Input: part model. Units: mm. Frame: model coordinates. Coordinates: 2 decimals unless noted, no trailing zeros. Loops run counter-clockwise (first coordinate to the right, second up) from the corner with the lowest first, then second, coordinate; pieces in that order, holes last. Notation, with made-up numbers: M 13,86.25 L 18,86.25 A28 cw 18,118.25 Z; hole C 61,38.5 d4. An arc over 180 degrees is marked long. Use a Markdown table: item, result. Add a question column.
1. Section A-A on y = 6.5. Output: boundary loops of the cut face in (x, z).
2. Section C-C on y = -4. Output: boundary loops of the cut face in (x, z).
3. Section B-B on x = -10.5. Output: boundary loops of the cut face in (y, z), then the cut area to 3 significant figures.
4. Pin query (flat end, axial travel): pin 1 (1.5 mm diameter, centred on x = 27, z = 0.5, fed in from +Y); pin 2 (1.5 mm diameter, centred on x = 27.5, z = 1, fed in from -Y); pin 3 (1.5 mm diameter, centred on y = -31, z = 2.5, fed in from -X); pin 4 (1.3 mm diameter, centred on x = 10.5, y = 0, fed in from -Z). Return the tip coordinate at first contact, or that it passes through.
5. Line query: L1, parallel to Y at x = -22.6, z = 1.95; L2, parallel to Y at x = 10.5, z = 0.95; L3, parallel to Y at x = -4, z = 2.9. Output: solid intervals per line, ascending. Write a range as [from, to].
6. Section D-D on y = -38.5. Output: boundary loops of the cut face in (x, z).
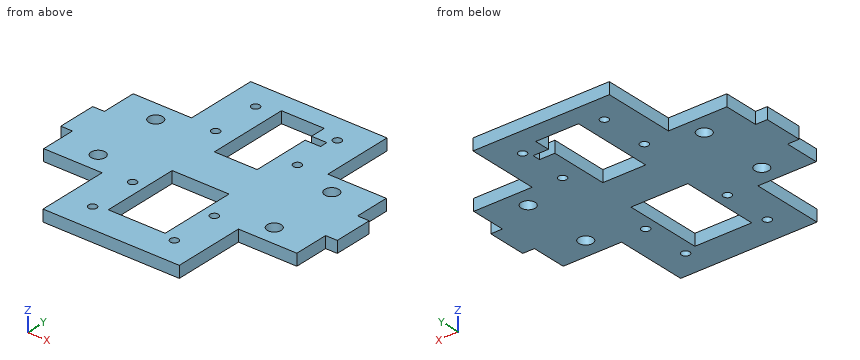
Autodesk Inventor part; units mm, degrees
ref_plane "YZ Plane" through (0, 0, 0) normal (1, 0, 0) x (0, 1, 0)
ref_plane "XZ Plane" through (0, 0, 0) normal (0, 1, 0) x (-1, 0, 0)
ref_plane "XY Plane" through (0, 0, 0) normal (0, 0, 1) x (1, 0, 0)
sketch "Sketch1" plane through (0, 0, 0) normal (0, 0, 1) x (1, 0, 0)
  line L0 (-17.5, 19.5) -> (17.5, 19.5)
  line L1 (17.5, 19.5) -> (17.5, -14.5)
  line L2 (17.5, -14.5) -> (-17.5, -14.5)
  line L3 (-17.5, -14.5) -> (-17.5, 19.5)
  line L4 (-12.5, 14.5) -> (-12.5, -9.5) construction
  line L5 (12.5, 14.5) -> (-12.5, 14.5) construction
  line L6 (12.5, -9.5) -> (12.5, 14.5) construction
  line L7 (-12.5, -9.5) -> (12.5, -9.5) construction
  line L8 (8.7, 9.1) -> (8.7, 9.9) construction
  line L9 (8.7, 9.9) -> (7.48, 9.9) construction
  line L10 (7.48, 9.9) -> (7.48, 9.1) construction
  line L11 (7.48, 9.1) -> (8.7, 9.1) construction
  circle A0 centre (-10.5, 12.5) radius 1.05
  circle A1 centre (-10.5, 0) radius 1.05
  circle A2 centre (10.5, 12.5) radius 1.05
  circle A3 centre (10.5, 0) radius 1.05
  line L12 (-5.5, 14.5) -> (-5.5, -6.5)
  line L13 (-5.5, -6.5) -> (5.5, -6.5)
  line L14 (5.5, -6.5) -> (5.5, 8.5)
  line L15 (5.5, 8.5) -> (9.45, 8.5)
  line L16 (9.45, 8.5) -> (9.45, 10.5)
  line L17 (9.45, 10.5) -> (5.5, 10.5)
  line L18 (5.5, 10.5) -> (5.5, 14.5)
  line L19 (-5.5, 14.5) -> (5.5, 14.5)
  point P0 (0, 0)
  dimension "d0" = 5
  dimension "d1" = 5
  dimension "d2" = 35
  dimension "d3" = 5
  dimension "d4" = 5
  dimension "d5" = 7
  dimension "d6" = 7
  dimension "d7" = 3
  dimension "d8" = 18
  dimension "d9" = 3.05
  dimension "d10" = 4
extrude "Extrusion1" add sketch "Sketch1" along normal blind 3
sketch "Sketch2" plane through (0, 0, 3) normal (0, 0, 1) x (1, 0, 0)
  line L0 (-17.5, -14.5) -> (17.5, -14.5) construction
  line L1 (-17.5, 19.5) -> (-17.5, -14.5) construction
  line L2 (17.5, -14.5) -> (17.5, 19.5) construction
  line L3 (-17.5, -14.5) -> (17.5, -14.5)
  line L4 (17.5, -14.5) -> (17.5, -45.5)
  line L5 (17.5, -45.5) -> (-17.5, -45.5)
  line L6 (-17.5, -45.5) -> (-17.5, -14.5)
  line L7 (-12.5, -16.5) -> (-12.5, -40.5) construction
  line L8 (12.5, -40.5) -> (12.5, -16.5) construction
  line L9 (12.5, -16.5) -> (-12.5, -16.5) construction
  line L10 (-12.5, -40.5) -> (12.5, -40.5) construction
  line L11 (-7.3, -17.5) -> (7.3, -17.5)
  line L12 (7.3, -17.5) -> (7.3, -37.5)
  line L13 (7.3, -37.5) -> (-7.3, -37.5)
  line L14 (-7.3, -37.5) -> (-7.3, -17.5)
  circle A0 centre (-10.5, -26) radius 1.05
  circle A1 centre (-10.5, -38.5) radius 1.05
  circle A2 centre (10.5, -26) radius 1.05
  circle A3 centre (10.5, -38.5) radius 1.05
  point P0 (0, 0)
  dimension "d13" = 5
  dimension "d14" = 1
  dimension "d15" = 5.2
  dimension "d16" = 5.2
  dimension "d17" = 3
extrude "Extrusion2" add sketch "Sketch2" against normal blind 3
sketch "Sketch3" plane through (0, 0, 3) normal (0, 0, 1) x (1, 0, 0)
  line L0 (17.5, 19.5) -> (17.5, -45.5)
  line L1 (-17.5, 19.5) -> (-17.5, -45.5)
  line L2 (-17.5, -45.5) -> (-17.5, 19.5) construction
  line L3 (-17.5, -13) -> (17.5, -13) construction
  line L4 (17.5, 19.5) -> (17.5, -45.5) construction
  line L5 (17.5, 1) -> (32.5, 1)
  line L6 (32.5, 1) -> (32.5, -27)
  line L7 (32.5, -27) -> (17.5, -27)
  line L8 (17.5, -27) -> (17.5, 1)
  line L9 (32.5, -8) -> (35.5, -8)
  line L10 (35.5, -8) -> (35.5, -18)
  line L11 (35.5, -18) -> (32.5, -18)
  line L12 (32.5, -18) -> (32.5, -8)
  line L13 (17.5, -13) -> (35.5, -13) construction
  point P0 (0, 0)
  dimension "d20" = 15
  dimension "d21" = 14
  dimension "d22" = 14
  dimension "d23" = 3
  dimension "d24" = 5
  dimension "d25" = 5
extrude "Extrusion3" add sketch "Sketch3" against normal blind 3
ref_plane "Work Plane1" through (0, 19.5, 3) normal (1, 0, 0) x (0, 0, -1)
mirror "Mirror1" about plane through (0, 19.5, 3) normal (1, 0, 0) of "Extrusion3"
sketch "Sketch4" plane through (0, 0, 3) normal (0, 0, 1) x (1, 0, 0)
  circle A0 centre (22.6, -4) radius 1.8
  circle A1 centre (22.6, -22) radius 1.8
  circle A2 centre (-22.6, -22) radius 1.8
  circle A3 centre (-22.6, -4) radius 1.8
  point P0 (0, 0)
extrude "Extrusion4" cut sketch "Sketch4" against normal blind 14.1125
properties part number "Camera holder plate"
Answers below:
| question | item | result |
|---|---|---|
| 1 | outline | M -17.5,0 L -5.5,0 L -5.5,3 L -17.5,3 Z; M 5.5,0 L 17.5,0 L 17.5,3 L 5.5,3 Z |
| 2 | outline | M -32.5,0 L -24.4,0 L -24.4,3 L -32.5,3 Z; M -20.8,0 L -5.5,0 L -5.5,3 L -20.8,3 Z; M 5.5,0 L 20.8,0 L 20.8,3 L 5.5,3 Z; M 24.4,0 L 32.5,0 L 32.5,3 L 24.4,3 Z |
| 3 | outline | M -45.5,0 L -39.55,0 L -39.55,3 L -45.5,3 Z; M -37.45,0 L -27.05,0 L -27.05,3 L -37.45,3 Z; M -24.95,0 L -1.05,0 L -1.05,3 L -24.95,3 Z; M 1.05,0 L 11.45,0 L 11.45,3 L 1.05,3 Z; M 13.55,0 L 19.5,0 L 19.5,3 L 13.55,3 Z |
| 3 | area | 170 mm² |
| 4 | pin 1 | stops at y = 1 |
| 4 | pin 2 | stops at y = -27 |
| 4 | pin 3 | stops at x = -17.5 |
| 4 | pin 4 | passes through |
| 5 | L1 | y = [-27, -23.8], [-20.2, -5.8], [-2.2, 1] |
| 5 | L2 | y = [-45.5, -39.55], [-37.45, -27.05], [-24.95, -1.05], [1.05, 11.45], [13.55, 19.5] |
| 5 | L3 | y = [-45.5, -37.5], [-17.5, -6.5], [14.5, 19.5] |
| 6 | outline | M -17.5,0 L -11.55,0 L -11.55,3 L -17.5,3 Z; M -9.45,0 L 9.45,0 L 9.45,3 L -9.45,3 Z; M 11.55,0 L 17.5,0 L 17.5,3 L 11.55,3 Z |
